Check sheet for the modelled part. Datum: model origin and axes. Units: mm. A direction names the side the tool comes from. Round coordinates to 2 decimals unless told otherwise and drop trailing zeros. Loops run counter-clockwise (first coordinate to the right, second up) from the corner with the lowest first, then second, coordinate; pieces in that order, holes last. Notation, with made-up numbers: (26, 58) - (31, 58) arc R15 cw to (31, 86) - close; hole circle Ø8 at (72.5, -39.75). An arc over 180 degrees is marked (long way). Put each result on its own line as item: value. Start each with the question number.
```python
from build123d import *

# Parameters (mm, degrees)
F1_DEPTH = 0.5
F3_DEPTH = 36
F4_DEPTH = 36
F5_DEPTH = 25
F7_DEPTH = 25
F8_DEPTH = 0.223


with BuildPart() as f1:
    # F0 (on Right) → F1 (new body)
    with BuildSketch(Plane.YZ):
        Polygon((-35.463306278, 10.7429168718), (-71.463306278, 10.7429168718), (-71.463306278, 8.9429168718), (-70.463306278, 8.9429168718), (-36.463306278, 8.9429168718), (-35.463306278, 8.9429168718), align=None)
    extrude(amount=F1_DEPTH)

    # F2 (on face) → F3 (join)
    with BuildSketch(Plane.XZ.offset(71.463306278)):
        Polygon((0.5, 8.9429168718), (0.8214285714, 8.9429168718), (0.5, 10.7429168718), align=None)
    extrude(amount=-F3_DEPTH)

    # F2 (on face) → F4 (join)
    with BuildSketch(Plane.XZ.offset(71.463306278)):
        Polygon((0, 10.7429168718), (0.5, 10.7429168718), (1, 10.7429168718), (0.5, 13.5429168718), (1, 13.5429168718), (0.5, 16.3429168718), (1, 16.3429168718), (0.5, 19.1429168718), (1, 19.1429168718), (0.5, 21.9429168718), (1, 21.9429168718), (0.5, 24.7429168718), (1, 24.7429168718), (0.5, 27.5429168718), (1, 27.5429168718), (0.5, 30.3429168718), (1, 30.3429168718), (0.5, 33.1429168718), (1, 33.1429168718), (0.5, 35.9429168718), (1, 35.9429168718), (0.5, 38.7429168718), (1, 38.7429168718), (0.5, 41.5429168718), (1, 41.5429168718), (0.5, 44.3429168718), (1, 44.3429168718), (0.5, 47.1429168718), (1, 47.1429168718), (0.5, 49.9429168718), (1, 49.9429168718), (0.5, 52.7429168718), (1, 52.7429168718), (0.6579817238, 54.6582192183), (0.5, 54.6582192183), (0, 54.6582192183), align=None)
    extrude(amount=-F4_DEPTH)

    # F0 (on Right) → F5 (cut)
    with BuildSketch(Plane.YZ):
        Polygon((-58.463306278, 36.9429168718), (-58.463306278, 35.9429168718), (-58.463306278, 33.1429168718), (-58.463306278, 30.3429168718), (-58.463306278, 27.5429168718), (-48.463306278, 27.5429168718), (-48.463306278, 30.3429168718), (-48.463306278, 33.1429168718), (-48.463306278, 35.9429168718), (-48.463306278, 36.9429168718), (-57.463306278, 36.9429168718), align=None)
    extrude(amount=F5_DEPTH, mode=Mode.SUBTRACT)

    # F6 (on face) → F7 (cut)
    with BuildSketch(Plane(origin=(0, 0, 0), x_dir=(0, -1, 0), z_dir=(-1, 0, 0))):
        Polygon((35.463306278, 54.6582192183), (35.463306278, 35.9216630459), (53.4756928682, 53.9652556181), (71.463306278, 36.0087513756), (71.463306278, 54.6582192183), align=None)
    extrude(amount=-F7_DEPTH, mode=Mode.SUBTRACT)

    # F8 (cut): a face of the model
    f8_faces = [f1.faces().sort_by_distance(p)[0] for p in [
        (0.4107142857, -53.463306278, 36.9429168718),
    ]]
    extrude(f8_faces, amount=-F8_DEPTH, mode=Mode.SUBTRACT)


solid = f1.part
```
Q1. Material ranges on line 1 (X direction, y = -49, z = 40); line 2 (Y direction, x = 0.15, z = 28.5); line 3 (Z direction, x = 0.2, y = -51), recorded low to high. Write a range as from..to.
Q2. Cross-section at A-A on x = 0.3. Enter the section's corners in (y, z).
Q3. Draft check along Z on faces 1 (the face through (0.382, -44.343, 44.817)), 2 (the face through (0.754, -53.627, 45.723)), 3 (the face through (0.4, -35.463, 22.6)). Enter one of: +Z half, -Z half, draft (parallel to the pull), parting line (faces both ways), or undercut.
Q4. Cross-section at D-D on z = 26. Enter the section's corners in (x, y).
Q5. Set-up check for faces 4 (the face through (0.753, -53.583, 48.523)), 5 (the face through (0.4, -71.463, 22.7)): record each of +Z, -Z, +X, -X, +Y, -Y from which the full face is reachable in a straight line by a thin tool's end or side.
Q6. Cross-section at C-C on z = 32.5. Enter the section's corners in (x, y), and give its area (3 significant figures).
Q7. Cross-section at B-B on y = -64. Enter the section's corners in (x, z), and give its area (3 significant figures).
Answer list:
1. line 1: x = 0..0.78
1. line 2: y = -71.46..-58.46, -48.46..-35.46
1. line 3: z = 8.94..27.54, 37.17..51.49
2. outline: (-71.46, 8.94) - (-35.46, 8.94) - (-35.46, 35.92) - (-53.48, 53.97) - (-71.46, 36.01) - close; hole (-58.46, 27.54) - (-48.46, 27.54) - (-48.46, 37.17) - (-58.46, 37.17) - close
3. face 1: +Z half
3. face 2: undercut
3. face 3: draft
4. outline: (0, -71.46) - (0.78, -71.46) - (0.78, -35.46) - (0, -35.46) - close
5. face 4: +X, +Y, -Y
5. face 5: +Z, -Z, +X, -X, -Y
6. outline: (0, -71.46) - (0.61, -71.46) - (0.61, -58.46) - (0, -58.46) - close; (0, -48.46) - (0.61, -48.46) - (0.61, -35.46) - (0, -35.46) - close
6. area: 16.0 mm2
7. outline: (0, 8.94) - (0.82, 8.94) - (0.5, 10.74) - (1, 10.74) - (0.5, 13.54) - (1, 13.54) - (0.5, 16.34) - (1, 16.34) - (0.5, 19.14) - (1, 19.14) - (0.5, 21.94) - (1, 21.94) - (0.5, 24.74) - (1, 24.74) - (0.5, 27.54) - (1, 27.54) - (0.5, 30.34) - (1, 30.34) - (0.5, 33.14) - (1, 33.14) - (0.5, 35.94) - (1, 35.94) - (0.5, 38.74) - (1, 38.74) - (0.5, 41.54) - (1, 41.54) - (0.66, 43.46) - (0, 43.46) - close
7. area: 25.9 mm2
